Geometry check sheet. Reference: the model listing, model coordinates, mm. A direction names the side the tool comes from. Give positions to 0.01 mm unless a question says otherwise; leave off trailing zeros. Order: outer loops, then holes, each group sorted by start corner. A loop starts at its lowest first (then second) coordinate and runs counter-clockwise, first axis right, second up. Notation, with made-up numbers: M -20.75,-10 L 31.25,-10 A7 cw 31.25,-4 Z; hole C -34.75,50 d8. An arc over 180 degrees is marked long. One line per question, with ' | ' between items. Start each with the question number.
from build123d import *

# Parameters (mm, degrees)
CROQUIS1_R              = 3
SALIENTE_EXTRUIR1_DEPTH = 3
SALIENTE_EXTRUIR2_START = -1.5
CROQUIS2_R              = 0.75
SALIENTE_EXTRUIR2_DEPTH = 1.5
CROQUIS3_R              = 2.4
CORTAR_EXTRUIR1_DEPTH   = 2


with BuildPart() as part:
    # Croquis1 → Saliente-Extruir1 (new body)
    with BuildSketch(Plane(origin=(0, 0, 0), x_dir=(1, 0, 0), z_dir=(0, 1, 0))):
        with Locations(Location((0, 0, 0), (0, 0, 270))):
            Circle(CROQUIS1_R)
    extrude(amount=SALIENTE_EXTRUIR1_DEPTH)

    # Croquis2 → Saliente-Extruir2 (add)
    with BuildSketch(Plane(origin=(0, 3, 0), x_dir=(1, 0, 0), z_dir=(0, 1, 0)).offset(SALIENTE_EXTRUIR2_START)):
        with BuildLine():
            Line((5.4375, 1.694430214), (0.75, 2.90473751))
            ThreePointArc((0.75, 2.90473751), (2.371708245, 1.837117307), (3, 0))
            ThreePointArc((3, 0), (2.371708245, -1.837117307), (0.75, -2.90473751))
            Line((0.75, -2.90473751), (5.4375, -1.694430214))
            ThreePointArc((5.4375, -1.694430214), (6.75, 0), (5.4375, 1.694430214))
        make_face()
        with Locations(Location((5, 0, 0), (0, 0, 270))):
            Circle(CROQUIS2_R, mode=Mode.SUBTRACT)
    extrude(amount=SALIENTE_EXTRUIR2_DEPTH)

    # Croquis3 → Cortar-Extruir1 (cut)
    with BuildSketch(Plane.XZ):
        with Locations(Location((0, 0, 0), (0, 0, 270))):
            Circle(CROQUIS3_R)
    extrude(amount=-CORTAR_EXTRUIR1_DEPTH, mode=Mode.SUBTRACT)


solid = part.part
Item 1: Cross-section at A-A, the plane y = 2.8. Record the cut outline in (x, z).
Item 2: Material ranges on line 1 along X through (y, z) = (1.45, 0); line 2 along X through (y, z) = (1.75, -0.5); line 3 along Y through (x, z) = (-0.5, 1.5), recorded low to high.
Item 3: Cross-section at D-D, the plane y = 1.9. Record the cut outline in (x, z), plus the area to 3 significant figures.
Item 4: Cross-section at C-C, the plane x = 0. Record the cut outline in (y, z), plus the area to 3 significant figures.
Item 5: Set-up check for faces 4 (the cylindrical face through (2.024, 0.986, -1.29)), 5 (the flat face through (3.1, 2.2, -2.3)): record each of +Z, -Z, +X, -X, +Y, -Y from which the full face is reachable in a straight line by a thin tool's end or side.
Item 6: Mould release check, pull along Z, two halves, no side actions. Record for faces 1 (the cylindrical face through (-2.93, 1.15, -0.65)), 2 (the flat face through (1, 3, 0)), 3 (the cylindrical face through (4.268, 2.24, -0.163)): released by +Z, released by -Z, zero draft, split by the parting line, or undercut.
Item 7: Depth check by flat-ended pin: pin 1 (1.5 mm diameter, centred on x = 3.5, y = 2, fed in from +Z); pin 2 (1.4 mm diameter, centred on x = 5, z = 0, fed in from -Y); pin 3 (1.5 mm diameter, centred on x = -1.5, z = -0.5, fed in from -Y). Enter the tip coordinate at first touch or a pass-through.
Item 8: Cross-section at B-B, the plane z = 0. Record the cut outline in (x, y), plus the area to 3 significant figures.
Outcome:
1) outline: M 0.75,-2.9 L 5.44,-1.69 A1.75 ccw 5.44,1.69 L 0.75,2.9 A3 ccw long Z; hole C 5,0 d1.5
2) line 1: x = -3 to -2.4, 2.4 to 3 | line 2: x = -2.96 to -2.35, 2.35 to 4.44, 5.56 to 6.68 | line 3: y = 2 to 3
3) outline: M 0.75,-2.9 L 5.44,-1.69 A1.75 ccw 5.44,1.69 L 0.75,2.9 A3 ccw long Z; hole C 0,0 d4.8; hole C 5,0 d1.5 | area: 23.6 mm²
4) outline: M 0,-3 L 3,-3 L 3,3 L 0,3 L 0,2.4 L 2,2.4 L 2,-2.4 L 0,-2.4 Z | area: 8.40 mm²
5) face 4: -Y | face 5: -Z, +X, +Y, -Y
6) face 1: split by the parting line | face 2: zero draft | face 3: undercut
7) pin 1: stops at z = 2.39 | pin 2: passes through | pin 3: stops at y = 2
8) outline: M -3,0 L -2.4,0 L -2.4,2 L 2.4,2 L 2.4,0 L 3,0 L 3,1.5 L 4.25,1.5 L 4.25,3 L -3,3 Z; M 5.75,1.5 L 6.75,1.5 L 6.75,3 L 5.75,3 Z | area: 11.8 mm²
